from build123d import *

# Parameters (mm, degrees)
SKETCH1_W           = 90
SKETCH1_H           = 8
BOSS_EXTRUDE1_DEPTH = 10
BOSS_EXTRUDE2_DEPTH = 10
SKETCH4_R           = 2
CUT_EXTRUDE1_DEPTH  = 11
FILLET1_R           = 10
SKETCH5_R           = 1.6
CUT_EXTRUDE2_DEPTH  = 11
LPATTERN1_COUNT     = 10
LPATTERN1_PITCH     = 10


with BuildPart() as part:
    # Sketch1 → Boss-Extrude1 (new body)
    with BuildSketch(Plane(origin=(0, 0, 0), x_dir=(1, 0, 0), z_dir=(0, 1, 0))):
        Rectangle(SKETCH1_W, SKETCH1_H)
    extrude(amount=BOSS_EXTRUDE1_DEPTH)

    # Sketch3 → Boss-Extrude2 (add)
    with BuildSketch(Plane(origin=(0, 0, 0), x_dir=(1, 0, 0), z_dir=(0, 1, 0))):
        with BuildLine():
            Line((-22.5, 43.000049343), (-22.5, 4))
            Line((-22.5, 4), (22.5, 4))
            Line((22.5, 4), (22.5, 43.000049343))
            ThreePointArc((22.5, 43.000049343), (0, 65.500049343), (-22.5, 43.000049343))
        make_face()
    extrude(amount=BOSS_EXTRUDE2_DEPTH)

    # Sketch4 → Cut-Extrude1 (cut, through all)
    with BuildSketch(Plane(origin=(0, 10, 0), x_dir=(1, 0, 0), z_dir=(0, 1, 0))):
        with Locations((-15.5885, 52.000074014)):
            Circle(SKETCH4_R)
        with Locations((15.5885, 52.000074014)):
            Circle(SKETCH4_R)
        with Locations((0, 25)):
            Circle(SKETCH4_R)
    extrude(amount=-CUT_EXTRUDE1_DEPTH, mode=Mode.SUBTRACT)

    # Fillet1
    fillet1_edges = [part.edges().sort_by_distance(p)[0] for p in [
        (22.5, 5, -4),
        (-22.5, 5, -4),
    ]]
    fillet(fillet1_edges, radius=FILLET1_R)

    # Sketch5 → Cut-Extrude2 (cut, through all)
    with BuildSketch(Plane(origin=(0, 10, 0), x_dir=(1, 0, 0), z_dir=(0, 1, 0))):
        with Locations((-40, 0)):
            Circle(SKETCH5_R)
    cut_extrude2 = extrude(amount=-CUT_EXTRUDE2_DEPTH, mode=Mode.SUBTRACT)

    # LPattern1: Cut-Extrude2 ×10
    with Locations(*[(i * LPATTERN1_PITCH, 0, 0) for i in range(1, LPATTERN1_COUNT)]):
        add(cut_extrude2, mode=Mode.SUBTRACT)


solid = part.part
Design review of the part built by this model. Coordinates are the model's own, in mm. A direction names the side the tool comes from. Round coordinates to 2 decimals unless told otherwise and drop trailing zeros. Write each loop counter-clockwise with the first axis right and the second up, starting at its lowest first coordinate (ties: lowest second). Pieces come first, ordered by that corner, then holes. Notation, with made-up numbers: (17.25, -36) -> (29.25, -36) arc R26 ccw to (29.25, -16) -> close; hole circle Ø1 at (83.5, 16). An arc over 180 degrees is marked (long way). One line per question, with ' | ' between items.
(1) Insertion check: P1, Ø2.5, axis at x = 10, z = 0, coming from the +Y side; P2, Ø5, axis at y = 4, z = -34, coming from the -X side; P3, Ø6, axis at y = 6, z = -9.5, coming from the +X side; P4, Ø3, axis at y = 8, z = -14.5, coming from the -X side. Each pin has a flat end and moves straight along its axis. Give the tip position at first contact, or say it passes through.
Result sheet:
P1: through | P2: x = -22.5 | P3: x = 25.89 | P4: x = -22.55
(2) Take a section at A-A, the plane x = 0. State the section outline as (y, z) points, and give its area (3 significant figures).
Result sheet:
outline: (0, -65.5) -> (10, -65.5) -> (10, -27) -> (0, -27) -> close; (0, -23) -> (10, -23) -> (10, -1.6) -> (0, -1.6) -> close; (0, 1.6) -> (10, 1.6) -> (10, 4) -> (0, 4) -> close | area: 623 mm2
(3) Take a section at C-C, the plane y = 4. State how many separate pieces and enclosed holes the cut face has, and give its area (3 significant figures).
Result sheet:
separate pieces: 1 | enclosed holes: 12 | area: 3,200 mm2
(4) Wall thickness on line 1 (Z direction, x = 0, y = 5.5); line 2 (Z direction, x = -40, y = 4.75); line 3 (X direction, y = 6.5, z = -17): over which ranges is each line inside the solid? List them lowest first. Write a range as [from, to].
Result sheet:
line 1: [-65.5, -27], [-23, -1.6], [1.6, 4] | line 2: [-4, -1.6], [1.6, 4] | line 3: [-22.5, 22.5]
(5) Draft analysis for pull direction Z (two halves, no side actions). For faces 1 (the flat face through (-1, 5, 4)), 2 (the flat face through (-39, 5, -4)), 3 (the cylindrical face through (-41.18, 5.07, -1.08)), 4 (the cylindrical face through (-1.18, 5.07, -1.08)), state which applies: released by +Z, released by -Z, zero draft, split by the parting line, or undercut.
Result sheet:
face 1: released by +Z | face 2: released by -Z | face 3: undercut | face 4: undercut
(6) Take a section at B-B, the plane x = -40. State the section outline as (y, z) points.
Result sheet:
outline: (0, -4) -> (10, -4) -> (10, -1.6) -> (0, -1.6) -> close; (0, 1.6) -> (10, 1.6) -> (10, 4) -> (0, 4) -> close
(7) Machinability: for faces 5 (the flat face through (39, 5, -4)), 6 (the cylindrical face through (-31.6, 5.07, -0.07)), 7 (the flat face through (-22.5, 5, -29)), which of the approach directions +Z, -Z, +X, -X, +Y, -Y give a long, thin tool a straight path to every point of the face, cutting with its end or side? Answer none if there is none.
Result sheet:
face 5: -Z, +X, +Y, -Y | face 6: +Y, -Y | face 7: -Z, -X, +Y, -Y
